Verification items for the finished model (mm, model axes). A direction names the side the tool comes from. Round coordinates to 2 decimals unless told otherwise and drop trailing zeros. Write each loop counter-clockwise with the first axis right and the second up, starting at its lowest first coordinate (ties: lowest second). Pieces come first, ordered by that corner, then holes. Notation, with made-up numbers: M -22.5,78 L 24.5,78 A13 cw 24.5,100 Z; hole C 77,83 d4. An arc over 180 degrees is marked long. Write each question's results on one line, items separated by ' | '.
Autodesk Inventor part; units mm, degrees
ref_plane "YZ Plane" through (0, 0, 0) normal (1, 0, 0) x (0, 1, 0)
ref_plane "XZ Plane" through (0, 0, 0) normal (0, 1, 0) x (-1, 0, 0)
ref_plane "XY Plane" through (0, 0, 0) normal (0, 0, 1) x (1, 0, 0)
sketch "Sketch1" plane through (0, 0, 0) normal (0, 0, 1) x (1, 0, 0)
  line L0 (0, 0) -> (18, 0)
  line L1 (18, 0) -> (18, 32)
  line L2 (18, 32) -> (0, 32)
  line L3 (0, 32) -> (0, 0)
  dimension "d0" = 18
  dimension "d1" = 32
extrude "base" add sketch "Sketch1" along normal blind 25
sketch "Sketch2" plane through (0, 0, 25) normal (0, 0, 1) x (1, 0, 0)
  line L0 (18, 32) -> (0, 32)
  line L1 (9, 32) -> (9, 0)
  line L2 (9, 16) -> (9, 27.5)
  line L3 (9, 16) -> (20.5, 16) construction
  line L4 (9, 27.5) -> (15.25, 27.5)
  line L5 (15.25, 27.5) -> (15.25, 4.5)
  line L6 (15.25, 4.5) -> (2.75, 4.5)
  line L7 (2.75, 4.5) -> (2.75, 27.5)
  line L8 (2.75, 27.5) -> (9, 27.5)
  line L9 (0, 0) -> (18, 0)
  dimension "d4" = 11.5
  dimension "d5" = 90
  dimension "d6" = 6.25
  dimension "d7" = 23
  dimension "d8" = 12.5
extrude "servo_place" cut sketch "Sketch2" against normal blind 18
sketch "Sketch4" plane through (0, 0, 0) normal (0, 0, -1) x (-1, 0, 0)
  line L0 (-18, 32) -> (0, 32)
  line L1 (-9, 32) -> (-9, 22)
  circle A0 centre (-9, 22) radius 5
  point P0 (0, 0)
  point P1 (-13, 32)
  point P2 (-5, 32)
  dimension "d18" = 10
  dimension "d19" = 10
extrude "attacher" add sketch "Sketch4" along normal blind 120
fillet "Fillet2" radius 4 1 edges at (14, 22, 0)
sketch "Sketch3" plane through (0, 0, 25) normal (0, 0, 1) x (1, 0, 0)
  line L0 (2.75, 27.5) -> (15.25, 27.5)
  line L1 (9, 27.5) -> (9, 30.3)
  circle A0 centre (9, 30.3) radius 1
  line L2 (15.25, 4.5) -> (2.75, 4.5)
  line L3 (9, 4.5) -> (9, 1.7)
  circle A1 centre (9, 1.7) radius 1
  point P0 (0, 0)
  dimension "d11" = 2.8
  dimension "d12" = 2
  dimension "d13" = 2.8
  dimension "d14" = 2
extrude "screws_servo" cut sketch "Sketch3" against normal through all
sketch "Sketch5" plane through (9, 22, -120) normal (0, 0, -1) x (-1, 0, 0)
  circle A0 centre (0, 0) radius 2.5
  point P0 (9, -22)
  dimension "d23" = 5
extrude "hole_bar_rigify" cut sketch "Sketch5" against normal through all
sketch "Sketch6" plane through (0, 0, 25) normal (0, 0, 1) x (1, 0, 0)
  line L0 (0, 32) -> (0, 0)
  line L1 (2.75, 27.5) -> (15.25, 27.5)
  line L2 (0, 32) -> (2.75, 32)
  line L3 (2.75, 32) -> (2.75, 27.5)
  line L4 (2.75, 27.5) -> (0, 27.5)
  line L5 (0, 27.5) -> (0, 32)
  line L6 (18, 32) -> (15.2563, 32)
  line L7 (15.2563, 32) -> (15.2563, 27.5)
  line L8 (15.2563, 27.5) -> (18, 27.5)
  line L9 (18, 27.5) -> (18, 32)
  line L10 (15.25, 27.5) -> (15.25, 4.5)
  line L11 (18, 0) -> (15.25, 0)
  line L12 (15.25, 0) -> (15.25, 4.5)
  line L13 (15.25, 4.5) -> (18, 4.5)
  line L14 (18, 4.5) -> (18, 0)
  line L15 (0, 0) -> (2.75, 0)
  line L16 (2.75, 0) -> (2.75, 4.5)
  line L17 (2.75, 4.5) -> (0, 4.5)
  line L18 (0, 4.5) -> (0, 0)
extrude "pilars_top" add sketch "Sketch6" along normal blind 20
sketch "Sketch9" plane through (0, 0, 45) normal (0, 0, 1) x (1, 0, 0)
  line L0 (0, 32) -> (0, 22)
  line L1 (18, 0) -> (18, 22)
  line L2 (0, 32) -> (18, 32)
  line L3 (18, 32) -> (18, 0)
  line L4 (18, 0) -> (0, 0)
  line L5 (0, 0) -> (0, 32)
  line L6 (18, 32) -> (36, 32)
  line L7 (36, 32) -> (36, 0)
  line L8 (36, 0) -> (18, 0)
  line L9 (0, 32) -> (-18, 32)
  line L10 (-18, 32) -> (-18, 0)
  line L11 (-18, 0) -> (0, 0)
  point P0 (0, 0)
  dimension "d39" = 18
  dimension "d40" = 18
extrude "base_top" add sketch "Sketch9" along normal blind 5
chamfer "Chamfer1" distance 18 angle 45 4 edges at (18, 2.25, 45) (18, 29.75, 45) (0, 2.25, 45) (0, 29.75, 45)
sketch "Sketch10" plane through (0, 0, 50) normal (0, 0, 1) x (1, 0, 0)
  circle A0 centre (9, 22) radius 2.5
  circle A1 centre (9, 22) radius 6
  point P0 (0, 0)
  dimension "d46" = 12
extrude "screw_hole" cut sketch "Sketch10" against normal blind 5 contours A0 | A1
sketch "Sketch11" plane through (0, 0, 50) normal (0, 0, 1) x (1, 0, 0)
  circle A0 centre (9, 22) radius 2.5
  line L0 (9, 22) -> (36, 22)
  line L1 (36, 4.5) -> (36, 27.5)
  line L2 (36, 22) -> (36, 24.5)
  line L3 (36, 24.5) -> (31, 24.5)
  line L4 (31, 24.5) -> (31, 19.5)
  line L5 (31, 19.5) -> (36, 19.5)
  line L6 (36, 22) -> (36, 19.5)
  line L7 (9, 22) -> (-18, 22)
  line L8 (-18, 27.5) -> (-18, 4.5)
  line L9 (-18, 22) -> (-18, 24.5)
  line L10 (-18, 24.5) -> (-13, 24.5)
  line L11 (-13, 24.5) -> (-13, 19.5)
  line L12 (-13, 19.5) -> (-18, 19.5)
  line L13 (-18, 19.5) -> (-18, 22)
  point P0 (0, 0)
  point P1 (36, 0)
  point P2 (36, 32)
  point P3 (-18, 32)
  point P4 (-18, 0)
  dimension "d49" = 2.5
  dimension "d50" = 5
  dimension "d51" = 5
  dimension "d52" = 2.5
  dimension "d53" = 5
  dimension "d54" = 5
extrude "Extrusion11" cut sketch "Sketch11" against normal blind 5 contours L11 L12 L8 L7 | L7 L8 L10 L11 | L4 L3 L1 L0 | L0 L1 L5 L4
properties part number "core_structure"
1) Depth check by flat-ended pin: P1, Ø1.2, axis at x = 9, y = 1.7, coming from the -Z side; P2, Ø10, axis at x = 27.5, z = 32, coming from the -Y side; P3, Ø6, axis at x = -10.5, z = 30.5, coming from the +Y side; P4, Ø5, axis at x = 2.5, z = -35.5, coming from the +Y side. Enter the tip coordinate at first touch or a pass-through.
Calculated:
P1: stops at z = 45 | P2: stops at y = 0 | P3: passes through | P4: stops at y = 25
2) Sectioned sample at A-A, the plane y = 22. Count the separate pieces of the cut face and the enclosed holes in it, and give its area (3 significant figures).
Calculated:
separate pieces: 4 | enclosed holes: 0 | area: 957 mm²
3) Draft check along X on faces 4 (the flat face through (18, 16, 13)), 5 (the flat face through (9, 13, 50)), 6 (the flat face through (2.75, 16, 16)), 7 (the flat face through (9, 4.5, 16)). Enter one of: pulls with the +X half, pulls with the -X half, needs draft (parallel to the pull), parting line crosses it, or undercut.
Calculated:
face 4: pulls with the +X half | face 5: needs draft | face 6: undercut | face 7: undercut
4) Sectioned sample at B-B, the plane y = 8. Record the cut outline in (x, z), and give its area (3 significant figures).
Calculated:
outline: M -18,45 L 36,45 L 36,50 L -18,50 Z; M 0,0 L 18,0 L 18,25 L 15.25,25 L 15.25,7 L 2.75,7 L 2.75,25 L 0,25 Z | area: 495 mm²
5) Sectioned sample at C-C, the plane z = 36. Record the cut outline in (x, y), and give its area (3 significant figures).
Calculated:
outline: M -9,0 L 2.75,0 L 2.75,4.5 L -9,4.5 Z; M -9,27.5 L 2.75,27.5 L 2.75,32 L -9,32 Z; M 15.25,0 L 27,0 L 27,4.5 L 15.25,4.5 Z; M 15.26,27.5 L 27,27.5 L 27,32 L 15.26,32 Z | area: 211 mm²
6) Sectioned sample at D-D, the plane z = -97.5. Record the cut outline in (x, y), and give its area (3 significant figures).
Calculated:
outline: C 9,22 d10; hole C 9,22 d5 | area: 58.9 mm²
7) Material ranges on line 1 (Z direction, x = 17, y = 10); line 2 (X direction, y = 30.3, z = 13.5); line 3 (Z direction, x = 9, y = 11.5), recorded low to high. Write a range as [from, to].
Calculated:
line 1: z = [0, 25], [45, 50] | line 2: x = [0, 8], [10, 18] | line 3: z = [0, 7], [45, 50]
8) Access from +Z, -Z, +X, -X, +Y, -Y to the whole of each face (thin tool, end or side, straight path). Record for faces 1 (the flat face through (34, 24.5, 48)), 2 (the flat face through (0, 16, 13)), 3 (the flat face through (9, 16, 7)).
Calculated:
face 1: +Z, -Z, +X | face 2: -Z, -X, +Y, -Y | face 3: none
